Geometry: final body of the model. Coordinates: model frame, mm. A direction names the side the tool comes from. Coordinates: 2 decimals unless noted, no trailing zeros. Loops run counter-clockwise (first coordinate to the right, second up) from the corner with the lowest first, then second, coordinate; pieces in that order, holes last. Notation, with made-up numbers: (45.5, -14.75) - (67.5, -14.75) arc R23 ccw to (67.5, 22.25) - close; hole circle Ø7 at (-30, 1.5). An arc over 180 degrees is marked (long way). Answer in a Markdown table with one row per item.
from build123d import *

# Parameters (mm, degrees)
SKETCH1_R           = 6.35
BOSS_EXTRUDE1_DEPTH = 6.096
BOSS_EXTRUDE2_DEPTH = 1.778
CUT_EXTRUDE1_START  = -1.778
CUT_EXTRUDE1_DEPTH  = 1.778
SKETCH5_R           = 6.35
BOSS_EXTRUDE3_DEPTH = 1.778
FILLET2_R           = 2.54
BOSS_EXTRUDE5_START = 3.81
BOSS_EXTRUDE5_DEPTH = 3.81
BOSS_EXTRUDE6_DEPTH = 5.08


with BuildPart() as part:
    # Sketch1 → Boss-Extrude1 (new body)
    with BuildSketch(Plane.XY):
        with Locations(Location((0, 0, 0), (0, 0, 180))):
            Circle(SKETCH1_R)
        with BuildLine():
            Line((-1.778, 2.155261469), (-1.778, -2.155261469))
            ThreePointArc((-1.778, -2.155261469), (0, -2.794), (1.778, -2.155261469))
            Line((1.778, -2.155261469), (1.778, 2.155261469))
            ThreePointArc((1.778, 2.155261469), (0, 2.794), (-1.778, 2.155261469))
        make_face(mode=Mode.SUBTRACT)
    extrude(amount=BOSS_EXTRUDE1_DEPTH)

    # Sketch3 → Boss-Extrude2 (add)
    with BuildSketch(Plane.XY.offset(3.81)):
        with BuildLine():
            Line((-6.35, 19.05), (6.35, 19.05))
            ThreePointArc((6.35, 19.05), (15.330256121, 15.330256121), (19.05, 6.35))
            Line((19.05, 6.35), (19.05, -6.35))
            ThreePointArc((19.05, -6.35), (15.330256121, -15.330256121), (6.35, -19.05))
            Line((6.35, -19.05), (-6.35, -19.05))
            ThreePointArc((-6.35, -19.05), (-15.330256121, -15.330256121), (-19.05, -6.35))
            Line((-19.05, -6.35), (-19.05, 6.35))
            ThreePointArc((-19.05, 6.35), (-15.330256121, 15.330256121), (-6.35, 19.05))
        make_face()
    extrude(amount=BOSS_EXTRUDE2_DEPTH)

    # Sketch4 → Cut-Extrude1 (cut)
    with BuildSketch(Plane.XY.offset(5.588).offset(CUT_EXTRUDE1_START)):
        with BuildLine():
            Line((-1.778, 2.155261469), (-1.778, -2.155261469))
            ThreePointArc((-1.778, -2.155261469), (0, -2.794), (1.778, -2.155261469))
            Line((1.778, -2.155261469), (1.778, 2.155261469))
            ThreePointArc((1.778, 2.155261469), (0, 2.794), (-1.778, 2.155261469))
        make_face()
    extrude(amount=CUT_EXTRUDE1_DEPTH, mode=Mode.SUBTRACT)

    # Sketch5 → Boss-Extrude3 (add)
    with BuildSketch(Plane.XY.offset(6.096)):
        with Locations(Location((0, 0, 0), (0, 0, 180))):
            Circle(SKETCH5_R)
    extrude(amount=BOSS_EXTRUDE3_DEPTH)

    # Fillet2
    # the kernel refuses this fillet: 2.54 mm, written as the material it takes off along each edge
    with BuildSketch(Plane(origin=(0, 0, 7.874), x_dir=(-1, 0, 0), z_dir=(0, 1, 0))) as fillet2_piece_1:
        with BuildLine():
            CenterArc((3.82273191, -2.54), FILLET2_R, 5.739170477, 84.260829523)
            Line((3.82273191, 0), (3.82273191, 0.0508))
            Line((3.82273191, 0.0508), (6.35, 0.0508))
            Line((6.35, 0.0508), (6.4008, 0))
            ThreePointArc((6.4008, 0), (6.4008, -1.143), (6.400545362, -2.28092))
            Line((6.400545362, -2.28092), (6.35, -2.286))
        make_face()
    revolve(axis=Axis((0, 0, 7.874), (0, 0, 1)), mode=Mode.SUBTRACT)

    # Sketch6 → Boss-Extrude5 (add)
    with BuildSketch(Plane(origin=(0, 0, 3.81), x_dir=(-1, 0, 0), z_dir=(0, 0, -1)).offset(BOSS_EXTRUDE5_START)):
        with BuildLine():
            Line((-6.35, 19.05), (6.35, 19.05))
            ThreePointArc((6.35, 19.05), (15.330256121, 15.330256121), (19.05, 6.35))
            Line((19.05, 6.35), (19.05, -6.35))
            ThreePointArc((19.05, -6.35), (15.330256121, -15.330256121), (6.35, -19.05))
            Line((6.35, -19.05), (-6.35, -19.05))
            ThreePointArc((-6.35, -19.05), (-15.330256121, -15.330256121), (-19.05, -6.35))
            Line((-19.05, -6.35), (-19.05, 6.35))
            ThreePointArc((-19.05, 6.35), (-15.330256121, 15.330256121), (-6.35, 19.05))
        make_face()
        with BuildLine():
            Line((-17.272, 6.35), (-17.272, -6.35))
            ThreePointArc((-17.272, -6.35), (-14.073020264, -14.073020264), (-6.35, -17.272))
            Line((-6.35, -17.272), (6.35, -17.272))
            ThreePointArc((6.35, -17.272), (14.073020264, -14.073020264), (17.272, -6.35))
            Line((17.272, -6.35), (17.272, 6.35))
            ThreePointArc((17.272, 6.35), (14.073020264, 14.073020264), (6.35, 17.272))
            Line((6.35, 17.272), (-6.35, 17.272))
            ThreePointArc((-6.35, 17.272), (-14.073020264, 14.073020264), (-17.272, 6.35))
        make_face(mode=Mode.SUBTRACT)
    extrude(amount=-BOSS_EXTRUDE5_DEPTH)

    # Sketch7 → Boss-Extrude6 (add)
    with BuildSketch(Plane.XY.offset(5.588)):
        with BuildLine():
            Line((-6.35, 17.018), (6.35, 17.018))
            ThreePointArc((6.35, 17.018), (13.893415142, 13.893415142), (17.018, 6.35))
            Line((17.018, 6.35), (17.018, -6.35))
            ThreePointArc((17.018, -6.35), (13.893415142, -13.893415142), (6.35, -17.018))
            Line((6.35, -17.018), (-6.35, -17.018))
            ThreePointArc((-6.35, -17.018), (-13.893415142, -13.893415142), (-17.018, -6.35))
            Line((-17.018, -6.35), (-17.018, 6.35))
            ThreePointArc((-17.018, 6.35), (-13.893415142, 13.893415142), (-6.35, 17.018))
        make_face()
        with BuildLine():
            ThreePointArc((-6.35, 15.24), (-12.636179285, 12.636179285), (-15.24, 6.35))
            Line((-15.24, 6.35), (-15.24, -6.35))
            ThreePointArc((-15.24, -6.35), (-12.636179285, -12.636179285), (-6.35, -15.24))
            Line((-6.35, -15.24), (6.35, -15.24))
            ThreePointArc((6.35, -15.24), (12.636179285, -12.636179285), (15.24, -6.35))
            Line((15.24, -6.35), (15.24, 6.35))
            ThreePointArc((15.24, 6.35), (12.636179285, 12.636179285), (6.35, 15.24))
            Line((6.35, 15.24), (-6.35, 15.24))
        make_face(mode=Mode.SUBTRACT)
    extrude(amount=BOSS_EXTRUDE6_DEPTH)


solid = part.part
(1) Cut plane C-C on x = 0. Output: boundary loops of the cut face in (y, z), then the cut area to 3 significant figures.
Verdict:
| item | result |
|---|---|
| outline | (-19.05, 0) - (-17.27, 0) - (-17.27, 3.81) - (-6.35, 3.81) - (-6.35, 0) - (-2.79, 0) - (-2.79, 6.1) - (2.79, 6.1) - (2.79, 0) - (6.35, 0) - (6.35, 3.81) - (17.27, 3.81) - (17.27, 0) - (19.05, 0) - (19.05, 5.59) - (17.02, 5.59) - (17.02, 10.67) - (15.24, 10.67) - (15.24, 5.59) - (6.35, 5.59) arc R2.54 ccw to (3.82, 7.87) - (-3.82, 7.87) arc R2.54 ccw to (-6.35, 5.59) - (-15.24, 5.59) - (-15.24, 10.67) - (-17.02, 10.67) - (-17.02, 5.59) - (-19.05, 5.59) - close |
| area | 140 mm² |
(2) Access query for faces 4 (the face through (13.81, 13.976, 8.092)), 5 (the face through (12.57, -12.7, 8.09)), 6 (the face through (0, 17.018, 8)), 7 (the face through (-17.272, 0, 2)), 8 (the face through (0, -17.018, 8)). Directions: +Z, -Z, +X, -X, +Y, -Y. A direction counts if a zero-diameter tool reaches every point of the face in a straight line with its end or side. Return the directions, or none.
Verdict:
| item | result |
|---|---|
| face 4 | +Z, +X, +Y |
| face 5 | +Z |
| face 6 | +Z, +X, -X, +Y |
| face 7 | -Z |
| face 8 | +Z, +X, -X, -Y |
(3) Cut plane A-A on z = 2.5. Output: boundary loops of the cut face in (x, y).
Verdict:
| item | result |
|---|---|
| outline | (-19.05, -6.35) arc R12.7 ccw to (-6.35, -19.05) - (6.35, -19.05) arc R12.7 ccw to (19.05, -6.35) - (19.05, 6.35) arc R12.7 ccw to (6.35, 19.05) - (-6.35, 19.05) arc R12.7 ccw to (-19.05, 6.35) - close; circle Ø12.7 at (0, 0); hole (-17.27, -6.35) arc R10.92 ccw to (-6.35, -17.27) - (6.35, -17.27) arc R10.92 ccw to (17.27, -6.35) - (17.27, 6.35) arc R10.92 ccw to (6.35, 17.27) - (-6.35, 17.27) arc R10.92 ccw to (-17.27, 6.35) - close; hole (-1.78, -2.16) arc R2.79 ccw to (1.78, -2.16) - (1.78, 2.16) arc R2.79 ccw to (-1.78, 2.16) - close |
(4) First-contact query: pin 1 Ø2.5 at (y, z) = (-2.5, 7) entering from -X; pin 2 Ø2.5 at (x, y) = (-0.5, 2) entering from +Z; pin 3 Ø1.8 at (x, y) = (0.5, 1.5) entering from -Z. Flat tips, straight axial feed; report the tip coordinate or a pass-through.
Verdict:
| item | result |
|---|---|
| pin 1 | stops at x = -17.02 |
| pin 2 | stops at z = 7.87 |
| pin 3 | stops at z = 6.1 |
(5) Ray query, probe 1 along X at (y, z) = (-1, 4.25); probe 2 along Y at (x, z) = (3, 0.75). Return the intervals inside material, ascending.
Verdict:
| item | result |
|---|---|
| probe 1 | x = -19.05 to -1.78, 1.78 to 19.05 |
| probe 2 | y = -19.05 to -17.27, -5.6 to 5.6, 17.27 to 19.05 |
(6) Cut plane B-B on y = 0. Output: boundary loops of the cut face in (x, z).
Verdict:
| item | result |
|---|---|
| outline | (-19.05, 0) - (-17.27, 0) - (-17.27, 3.81) - (-6.35, 3.81) - (-6.35, 0) - (-1.78, 0) - (-1.78, 6.1) - (1.78, 6.1) - (1.78, 0) - (6.35, 0) - (6.35, 3.81) - (17.27, 3.81) - (17.27, 0) - (19.05, 0) - (19.05, 5.59) - (17.02, 5.59) - (17.02, 10.67) - (15.24, 10.67) - (15.24, 5.59) - (6.35, 5.59) arc R2.54 ccw to (3.82, 7.87) - (-3.82, 7.87) arc R2.54 ccw to (-6.35, 5.59) - (-15.24, 5.59) - (-15.24, 10.67) - (-17.02, 10.67) - (-17.02, 5.59) - (-19.05, 5.59) - close |
(7) Cut plane D-D on x = -10. Output: boundary loops of the cut face in (y, z), then the cut area to 3 significant figures.
Verdict:
| item | result |
|---|---|
| outline | (-18.51, 0) - (-16.64, 0) - (-16.64, 3.81) - (16.64, 3.81) - (16.64, 0) - (18.51, 0) - (18.51, 5.59) - (16.37, 5.59) - (16.37, 10.67) - (14.46, 10.67) - (14.46, 5.59) - (-14.46, 5.59) - (-14.46, 10.67) - (-16.37, 10.67) - (-16.37, 5.59) - (-18.51, 5.59) - close |
| area | 99.6 mm² |
(8) Pull-direction query (X, two-part tool) for faces 1 (the face through (-15.43, -15.23, 2.75)), 2 (the face through (15.23, -15.43, 2.75)), 3 (the face through (12.7, 12.57, 8.09)); classes: pulls with the +X half, pulls with the -X half, needs draft (parallel to the pull), parting line crosses it, or undercut.
Verdict:
| item | result |
|---|---|
| face 1 | pulls with the -X half |
| face 2 | pulls with the +X half |
| face 3 | undercut |
